from build123d import *

# Parameters (mm, degrees)
SKETCH1_W                      = 40
SKETCH1_H                      = 20
BOSS_EXTRUDE1_DEPTH            = 12
CBORE_FOR_M5_SHCS1_D           = 5.5
CBORE_FOR_M5_SHCS1_DEPTH       = 12
CBORE_FOR_M5_SHCS1_CBORE_D     = 10.5
CBORE_FOR_M5_SHCS1_CBORE_DEPTH = 6
BOSS_EXTRUDE2_DEPTH            = 20
BOSS_EXTRUDE2_DEPTH_BACK       = 12
SKETCH6_R                      = 2.5
CUT_EXTRUDE1_DEPTH             = 14.25
CUT_EXTRUDE1_DEPTH_BACK        = 14.25
FILLET1_R                      = 4


with BuildPart() as part:
    # Sketch1 → Boss-Extrude1 (new body)
    with BuildSketch(Plane(origin=(0, 0, 0), x_dir=(1, 0, 0), z_dir=(0, 1, 0))):
        Rectangle(SKETCH1_W, SKETCH1_H)
    extrude(amount=BOSS_EXTRUDE1_DEPTH)

    # CBORE for M5 SHCS1
    with Locations(Plane(origin=(0, 12, 0), x_dir=(1, 0, 0), z_dir=(0, 1, 0))):
        with Locations((10, 0), (-10, 0)):
            CounterBoreHole(CBORE_FOR_M5_SHCS1_D / 2, CBORE_FOR_M5_SHCS1_CBORE_D / 2, CBORE_FOR_M5_SHCS1_CBORE_DEPTH, depth=CBORE_FOR_M5_SHCS1_DEPTH)

    # Sketch4 → Boss-Extrude2 (add, two sides)
    with BuildSketch(Plane(origin=(0, 12, 0), x_dir=(1, 0, 0), z_dir=(0, 1, 0))) as boss_extrude2_sk:
        with BuildLine():
            ThreePointArc((-12.4, -4.669314725), (0, -13.25), (12.4, -4.669314725))
            ThreePointArc((12.4, -4.669314725), (9.665081865, -5.239306237), (7.025, -4.325722483))
            ThreePointArc((7.025, -4.325722483), (0, -8.25), (-7.025, -4.325722483))
            ThreePointArc((-7.025, -4.325722483), (-9.665081865, -5.239306237), (-12.4, -4.669314725))
        make_face()
        with BuildLine():
            ThreePointArc((-7.025, 4.325722483), (-9.665081865, 5.239306237), (-12.4, 4.669314725))
            ThreePointArc((-12.4, 4.669314725), (0, 13.25), (12.4, 4.669314725))
            ThreePointArc((12.4, 4.669314725), (9.665081865, 5.239306237), (7.025, 4.325722483))
            ThreePointArc((7.025, 4.325722483), (0, 8.25), (-7.025, 4.325722483))
        make_face()
    extrude(amount=BOSS_EXTRUDE2_DEPTH)
    extrude(boss_extrude2_sk.sketch, amount=-BOSS_EXTRUDE2_DEPTH_BACK)

    # Sketch6 → Cut-Extrude1 (cut, two sides)
    with BuildSketch(Plane.XY) as cut_extrude1_sk:
        with Locations((0, 24.5)):
            Circle(SKETCH6_R)
    extrude(amount=CUT_EXTRUDE1_DEPTH, mode=Mode.SUBTRACT)
    extrude(cut_extrude1_sk.sketch, amount=-CUT_EXTRUDE1_DEPTH_BACK, mode=Mode.SUBTRACT)

    # Fillet1
    fillet1_edges = [part.edges().sort_by_distance(p)[0] for p in [
        (-20, 12, 0),
        (20, 12, 0),
    ]]
    fillet(fillet1_edges, radius=FILLET1_R)


solid = part.part
Source: CAD feature listing. Evaluate the final solid. Frame: model axes, mm. A direction names the side the tool comes from. Give positions to 0.01 mm unless a question says otherwise; leave off trailing zeros. Order: outer loops, then holes, each group sorted by start corner. A loop starts at its lowest first (then second) coordinate and runs counter-clockwise, first axis right, second up. Notation, with made-up numbers: (1.5, 72) -> (28.5, 72) arc R8 cw to (28.5, 78) -> close; hole circle Ø3 at (-26.75, 7). An arc over 180 degrees is marked (long way). Use a Markdown table: item, result.
1) Reachability of faces 1 (the flat face through (14, 6, -10)), 2 (the cylindrical face through (-0.22, 16.22, -13.25)), 3 (the cylindrical face through (-0.22, 16.22, 13.25)) from +Z, -Z, +X, -X, +Y, -Y: full face, straight path, thin tool, end or side. Return the list, or none.
Answer list:
| item | result |
|---|---|
| face 1 | -Z, +X, +Y, -Y |
| face 2 | -Z, +Y |
| face 3 | +Z, +Y |
2) Section query D-D, the plane x = 0. Return the cut outline in (y, z).
Answer list:
| item | result |
|---|---|
| outline | (0, -13.25) -> (22, -13.25) -> (22, -8.25) -> (12, -8.25) -> (12, 8.25) -> (22, 8.25) -> (22, 13.25) -> (0, 13.25) -> close; (27, -13.25) -> (32, -13.25) -> (32, -8.25) -> (27, -8.25) -> close; (27, 8.25) -> (32, 8.25) -> (32, 13.25) -> (27, 13.25) -> close |
3) Section query C-C, the plane y = 4. Return the cut outline in (x, z), then the cut area to 3 significant figures.
Answer list:
| item | result |
|---|---|
| outline | (-20, -10) -> (-8.69, -10) arc R13.25 ccw to (8.69, -10) -> (20, -10) -> (20, 10) -> (8.69, 10) arc R13.25 ccw to (-8.69, 10) -> (-20, 10) -> close; hole circle Ø5.5 at (-10, 0); hole circle Ø5.5 at (10, 0) |
| area | 830 mm² |
4) Section query A-A, the plane z = 0. Return the cut outline in (x, y).
Answer list:
| item | result |
|---|---|
| outline | (-20, 0) -> (-12.75, 0) -> (-12.75, 6) -> (-15.25, 6) -> (-15.25, 12) -> (-16, 12) arc R4 ccw to (-20, 8) -> close; (-7.25, 0) -> (7.25, 0) -> (7.25, 6) -> (4.75, 6) -> (4.75, 12) -> (-4.75, 12) -> (-4.75, 6) -> (-7.25, 6) -> close; (12.75, 0) -> (20, 0) -> (20, 8) arc R4 ccw to (16, 12) -> (15.25, 12) -> (15.25, 6) -> (12.75, 6) -> close |
5) Contact query for flat-ended pins moving along their axis: P1, Ø12, axis at y = 16.5, z = -2, coming from the -X side; P2, Ø6.5, axis at x = 10, z = 0, coming from the +Y side; P3, Ø2, axis at x = 14, z = 4, coming from the +Y side. Output: stop coordinate, or through.
Answer list:
| item | result |
|---|---|
| P1 | x = -19.12 |
| P2 | y = 6 |
| P3 | y = 12 |
6) Section query B-B, the plane x = 10. Return the cut outline in (y, z), then the cut area to 3 significant figures.
Answer list:
| item | result |
|---|---|
| outline | (0, -10) -> (12, -10) -> (12, -8.69) -> (32, -8.69) -> (32, -5.25) -> (6, -5.25) -> (6, -2.75) -> (0, -2.75) -> close; (0, 2.75) -> (6, 2.75) -> (6, 5.25) -> (32, 5.25) -> (32, 8.69) -> (12, 8.69) -> (12, 10) -> (0, 10) -> close |
| area | 282 mm² |
7) Mould query, pull axis Y, two halves, no side actions, for faces 4 (the flat face through (-14, 6, 10)), 5 (the cylindrical face through (18.859, 10.797, -0.14)), 6 (the cylindrical face through (-2.5, 24.6, 10.5)). Classes: +Y half, -Y half, draft (parallel to the pull), parting line (faces both ways), or undercut.
Answer list:
| item | result |
|---|---|
| face 4 | draft |
| face 5 | +Y half |
| face 6 | undercut |
8) Ray query, line 1 along Y through (x, z) = (0, 9.25); line 2 along Z through (x, y) = (-10, 2); line 3 along X through (y, z) = (5, -2.5). Return the intervals inside material, ascending. Write a range as [from, to].
Answer list:
| item | result |
|---|---|
| line 1 | [0, 22], [27, 32] |
| line 2 | [-10, -2.75], [2.75, 10] |
| line 3 | [-20, -11.15], [-8.85, 8.85], [11.15, 20] |
